Geometry check sheet. Reference: drawing and pictorial views, mm from the part's lowest x, y, z. A direction names the side the tool comes from. Give positions to 0.01 mm unless a question says otherwise; leave off trailing zeros. Write each loop counter-clockwise with the first axis right and the second up, starting at its lowest first coordinate (ties: lowest second). Pieces come first, ordered by that corner, then holes. Notation, with made-up numbers: (-8.5, -32) -> (8.5, -32) arc R13 cw to (8.5, -11) -> close; hole circle Ø2 at (-8.5, 29.25). An arc over 180 degrees is marked (long way). Use a Markdown table: item, result. Add a question column.
1. Set-up check for the marked faces 5 and 6: record each of +Z, -Z, +X, -X, +Y, -Y from which the full face is reachable in a straight line by a thin tool's end or side.
2. Release check for a two-part mould opening along Y. For the marked faces 1, 2, 3 and 4 record: released by +Y, released by -Y, zero draft, split by the parting line, or undercut.
3. Cross-section at D-D (y = 8.75). Enter the section's corners in (x, z), then the cut area to 3 significant figures.
4. Scan lines: probe 1 along Y at (x, z) = (2.75, 2); probe 2 along X at (y, z) = (2.5, 7.25); probe 3 along X at (y, z) = (6.75, 3). Record each from-to range of solid material in increasing order. Write a range as [from, to].
5. Cross-section at C-C (z = 1). Enter the section's corners in (x, y).
6. Cross-section at A-A (z = 8). Enter the section's corners in (x, y), then the cut area to 3 significant figures.
7. Cross-section at B-B (x = 26.25). Enter the section's corners in (y, z), then the cut area to 3 significant figures.
8. Gauge pin test, flat ends, axial feed: P1, Ø3, axis at x = 18, z = 7.5, coming from the -Y side; P2, Ø5, axis at x = 23, z = 2.5, coming from the -Y side. Record the tip position at first contact, or that the pin passes through.
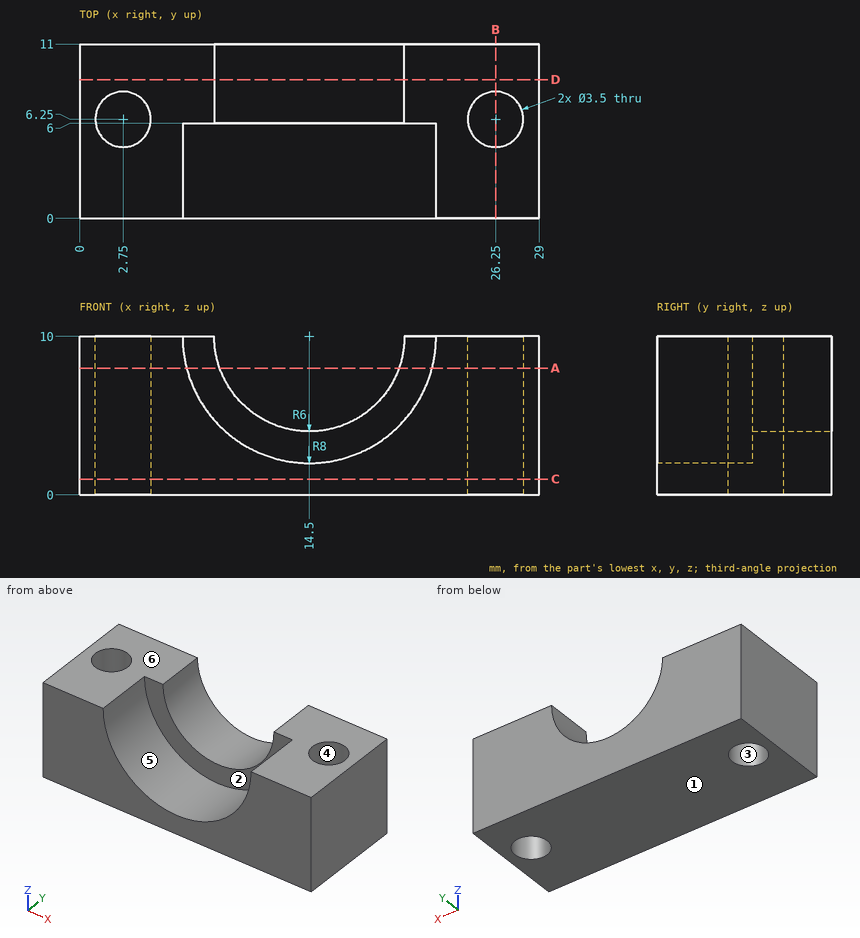
Worked answers:
| question | item | result |
|---|---|---|
| 1 | face 5 | +Z, -Y |
| 1 | face 6 | +Z, +X, -X, +Y, -Y |
| 2 | face 1 | zero draft |
| 2 | face 2 | released by -Y |
| 2 | face 3 | undercut |
| 2 | face 4 | undercut |
| 3 | outline | (0, 0) -> (29, 0) -> (29, 10) -> (20.5, 10) arc R6 cw to (8.5, 10) -> (0, 10) -> close |
| 3 | area | 233 mm² |
| 4 | probe 1 | y = [0, 4.5], [8, 11] |
| 4 | probe 2 | x = [0, 6.99], [22.01, 29] |
| 4 | probe 3 | x = [0, 1.07], [4.43, 24.57], [27.93, 29] |
| 5 | outline | (0, 0) -> (29, 0) -> (29, 11) -> (0, 11) -> close; hole circle Ø3.5 at (2.75, 6.25); hole circle Ø3.5 at (26.25, 6.25) |
| 6 | outline | (0, 0) -> (6.75, 0) -> (6.75, 6) -> (8.84, 6) -> (8.84, 11) -> (0, 11) -> close; (20.16, 6) -> (22.25, 6) -> (22.25, 0) -> (29, 0) -> (29, 11) -> (20.16, 11) -> close; hole circle Ø3.5 at (2.75, 6.25); hole circle Ø3.5 at (26.25, 6.25) |
| 6 | area | 150 mm² |
| 7 | outline | (0, 0) -> (4.5, 0) -> (4.5, 10) -> (0, 10) -> close; (8, 0) -> (11, 0) -> (11, 10) -> (8, 10) -> close |
| 7 | area | 75.0 mm² |
| 8 | P1 | passes through |
| 8 | P2 | stops at y = 0 |
